Input: part model. Units: mm. Frame: model coordinates. Give positions to 0.01 mm unless a question says otherwise; leave off trailing zeros. Loops run counter-clockwise (first coordinate to the right, second up) from the corner with the lowest first, then second, coordinate; pieces in that order, holes last. Notation, with made-up numbers: (-33.75, 2.5) - (6.25, 2.5) arc R21 cw to (6.25, 25.5) - close; hole circle Ø7 at (84, -10.75). An arc over 180 degrees is marked (long way). Answer as a JSON object with one key per item and string values. Group by question number.
(1) Mould query, pull axis X, two halves, no side actions, for faces 1 (the cylindrical face through (9.125, 0.789, -14.361)), 2 (the flat face through (6.78, 1, -7)), 3 (the flat face through (18, 1, 1.38)). Classes: +X half, -X half, draft (parallel to the pull), parting line (faces both ways), or undercut.
(2) Section query C-C (x = 26.76). Return loops of the section in (y, z), plus the area to 3 significant figures.
(3) Section query B-B (z = -5.42). Return loops of the section in (x, y), plus the area to 3 significant figures.
(4) Material intervals for L1, parallel to Z at x = 24.73, y = 0.75; L2, parallel to X at y = 1.25, z = 0; L3, parallel to X at y = 0.8, z = -9.82, sorted ascending.
(5) Pin query (flat end, axial travel): P1, Ø1.6, axis at x = 26.76, z = 0, coming from the -Y side; P2, Ø2, axis at x = 9.32, z = -15.24, coming from the +Y side. Return the tip coordinate at first contact, or that it passes through.
(6) Section query A-A (y = 0.95). Return loops of the section in (x, z), plus the area to 3 significant figures.
```python
from build123d import *

# Parameters (mm, degrees)
SKETCH1_W           = 22
SKETCH1_H           = 18
BOSS_EXTRUDE2_DEPTH = 1.6
SKETCH4_R           = 0.9
CUT_EXTRUDE5_DEPTH  = 1.6
SKETCH9_R           = 0.4
CUT_EXTRUDE6_DEPTH  = 10


with BuildPart() as part:
    # Sketch1 → Boss-Extrude2 (new body)
    with BuildSketch(Plane(origin=(0, 0, 0), x_dir=(1, 0, 0), z_dir=(0, 1, 0))):
        with Locations((17.78, 7.62)):
            Rectangle(SKETCH1_W, SKETCH1_H)
    extrude(amount=BOSS_EXTRUDE2_DEPTH)

    # Sketch4 → Cut-Extrude5 (cut)
    with BuildSketch(Plane(origin=(0, 0, 0), x_dir=(1, 0, 0), z_dir=(0, 1, 0))):
        with Locations((26.76, 15.24)):
            Circle(SKETCH4_R)
        with Locations((26.76, 0)):
            Circle(SKETCH4_R)
        with Locations((9.32, 0)):
            Circle(SKETCH4_R)
        with Locations((9.32, 15.24)):
            Circle(SKETCH4_R)
    extrude(amount=CUT_EXTRUDE5_DEPTH, mode=Mode.SUBTRACT)

    # Sketch9 → Cut-Extrude6 (cut)
    with BuildSketch(Plane(origin=(0, 0, 0), x_dir=(1, 0, 0), z_dir=(0, 1, 0))):
        with Locations((24.73, 5.42)):
            Circle(SKETCH9_R)
        with Locations((24.73, 9.82)):
            Circle(SKETCH9_R)
    extrude(amount=CUT_EXTRUDE6_DEPTH, mode=Mode.SUBTRACT)


solid = part.part
```
Recorded:
{
 "1": {"face 1": "undercut", "face 2": "-X half", "face 3": "draft"},
 "2": {"outline": "(0, -16.62) - (1.6, -16.62) - (1.6, -16.14) - (0, -16.14) - close; (0, -14.34) - (1.6, -14.34) - (1.6, -0.9) - (0, -0.9) - close; (0, 0.9) - (1.6, 0.9) - (1.6, 1.38) - (0, 1.38) - close", "area": "23.0 mm^2"},
 "3": {"outline": "(6.78, 0) - (24.33, 0) - (24.33, 1.6) - (6.78, 1.6) - close; (25.13, 0) - (28.78, 0) - (28.78, 1.6) - (25.13, 1.6) - close", "area": "33.9 mm^2"},
 "4": {"L1": "z = -16.62 to -10.22, -9.42 to -5.82, -5.02 to 1.38", "L2": "x = 6.78 to 8.42, 10.22 to 25.86, 27.66 to 28.78", "L3": "x = 6.78 to 24.33, 25.13 to 28.78"},
 "5": {"P1": "passes through", "P2": "stops at y = 1.6"},
 "6": {"outline": "(6.78, -16.62) - (28.78, -16.62) - (28.78, 1.38) - (6.78, 1.38) - close; hole circle Ø1.8 at (9.32, -15.24); hole circle Ø1.8 at (9.32, 0); hole circle Ø0.8 at (24.73, -9.82); hole circle Ø0.8 at (24.73, -5.42); hole circle Ø1.8 at (26.76, -15.24); hole circle Ø1.8 at (26.76, 0)", "area": "385 mm^2"}
}
